```python
from build123d import *

# Parameters (mm, degrees)
CYLINDER006_R     = 2.1
CYLINDER006_DEPTH = 20
SKETCH005_R       = 2.1
EXTRUDE004_DEPTH  = 10
BOX003_W          = 8
BOX003_H          = 55
BOX003_DEPTH      = 9
FILLET001_R       = 3


with BuildPart() as obj1:
    # Cylinder006 → Cylinder006 (new body)
    with BuildSketch(Plane(origin=(14.5, 23.2, -10), x_dir=(1, 0, 0), z_dir=(0, 0, 1))):
        Circle(CYLINDER006_R)
    extrude(amount=CYLINDER006_DEPTH)


with BuildPart() as obj2:
    # Sketch005 (on Face2 of Box003) → Extrude004 (new body)
    with BuildSketch(Plane(origin=(18.2, 17.6, -2.4), x_dir=(0, -1, 0), z_dir=(-1, 0, 0))):
        with Locations((3.8, 3.8)):
            Circle(SKETCH005_R)
        with Locations((39.8, 3.8)):
            Circle(SKETCH005_R)
    extrude(amount=EXTRUDE004_DEPTH)

    # Fusion006: union obj1
    add(obj1.part)


with BuildPart() as obj3:
    # Box003 → Box003 (new body)
    with BuildSketch(Plane(origin=(10.2, -26, -2.4), x_dir=(1, 0, 0), z_dir=(0, 0, 1))):
        with Locations((4, 27.5)):
            Rectangle(BOX003_W, BOX003_H)
    extrude(amount=BOX003_DEPTH)

    # Fillet001
    fillet001_edges = [obj3.edges().sort_by_distance(p)[0] for p in [
        (14.2, -26, -2.4),
        (14.2, -26, 6.6),
        (14.2, 29, -2.4),
    ]]
    fillet(fillet001_edges, radius=FILLET001_R)

    # Cut003: cut obj2
    add(obj2.part, mode=Mode.SUBTRACT)


solid = obj3.part
```
Work out the finished part from the listing and answer in its coordinate system (mm). Give positions to 0.01 mm unless a question says otherwise; leave off trailing zeros. Write each loop counter-clockwise with the first axis right and the second up, starting at its lowest first coordinate (ties: lowest second). Pieces come first, ordered by that corner, then holes. Notation, with made-up numbers: (74, 31.25) -> (123, 31.25) arc R24 cw to (123, 49.25) -> close; hole circle Ø7 at (70.25, 74). An arc over 180 degrees is marked (long way). Write item = value, one per line.
Q1. Section C-C on z = 2.5 is taken. Determine the outline of the cut face in (x, y).
Computed values:
outline = (10.2, -26) -> (18.2, -26) -> (18.2, -23.99) -> (10.2, -23.99) -> close; (10.2, -20.41) -> (18.2, -20.41) -> (18.2, 12.01) -> (10.2, 12.01) -> close; (10.2, 15.59) -> (18.2, 15.59) -> (18.2, 29) -> (10.2, 29) -> close; hole circle Ø4.2 at (14.5, 23.2)
Q2. A flat-ended cylindrical pin translates along its axis: pin 1 Ø1 at (x, z) = (17, -1) entering from -Y. Find the tip coordinate at first contact, or state that the pin passes through.
Computed values:
pin_1 = -25.79
Q3. Section A-A on x = 14.5 is taken. Determine the outline of the cut face in (y, z).
Computed values:
outline = (-26, 0.6) arc R3 ccw to (-23, -2.4) -> (21.1, -2.4) -> (21.1, 6.6) -> (-23, 6.6) arc R3 ccw to (-26, 3.6) -> close; (25.3, -2.4) -> (26, -2.4) arc R3 ccw to (29, 0.6) -> (29, 6.6) -> (25.3, 6.6) -> close; hole circle Ø4.2 at (-22.2, 1.4); hole circle Ø4.2 at (13.8, 1.4)
Q4. Section B-B on y = 23.2 is taken. Determine the outline of the cut face in (x, z), and give its area (3 significant figures).
Computed values:
outline = (10.2, -2.4) -> (12.4, -2.4) -> (12.4, 6.6) -> (10.2, 6.6) -> close; (16.6, -2.4) -> (18.2, -2.4) -> (18.2, 6.6) -> (16.6, 6.6) -> close
area = 34.2 mm^2
Q5. For a pull along Z with two mould halves and no side action, classify faces 1 (the cylindrical face through (14.26, 15.9, 1.49)), 2 (the flat face through (14, -26, 2)), 3 (the flat face through (14, 3, 6.6)), 4 (the flat face through (14, 2, -2.4)) as pulls with the +Z half, pulls with the -Z half, needs draft (parallel to the pull), parting line crosses it, or undercut.
Computed values:
face_1 = undercut
face_2 = needs draft
face_3 = pulls with the +Z half
face_4 = pulls with the -Z half
Q6. Consider line 1 along Z through (x, y) = (16.25, 13.8); line 2 along Y through (x, z) = (16.25, 1.4); line 3 along X through (y, z) = (23.2, 2). Determine where each line is inside the solid, lowest interval first.
Computed values:
line_1 = -2.4 to -0.7, 3.5 to 6.6
line_2 = -26 to -24.3, -20.1 to 11.7, 15.9 to 22.04, 24.36 to 29
line_3 = 10.2 to 12.4, 16.6 to 18.2
Q7. Section D-D on x = 17.5 is taken. Determine the outline of the cut face in (y, z).
Computed values:
outline = (-26, 0.6) arc R3 ccw to (-23, -2.4) -> (26, -2.4) arc R3 ccw to (29, 0.6) -> (29, 6.6) -> (-23, 6.6) arc R3 ccw to (-26, 3.6) -> close; hole circle Ø4.2 at (-22.2, 1.4); hole circle Ø4.2 at (13.8, 1.4)
